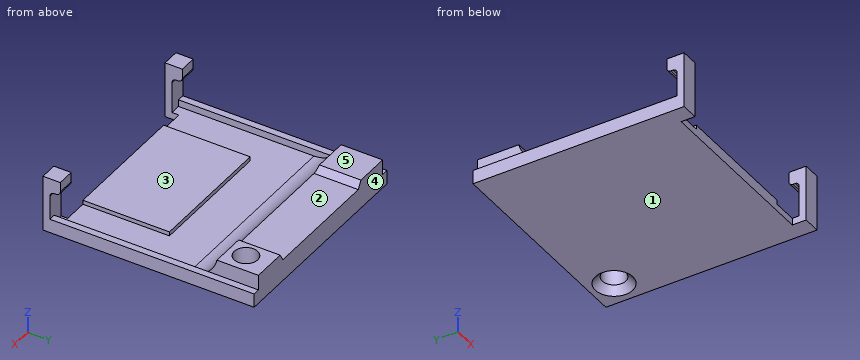
```python
from build123d import *

# Parameters (mm, degrees)
ESQUISSE1_W             = 28.6
ESQUISSE1_H             = 16.5
BOSS_EXTRU_1_DEPTH      = 1
ESQUISSE2_W             = 18.6
ESQUISSE2_H             = 12.5
BOSS_EXTRU_2_DEPTH      = 0.6
ESQUISSE3_W             = 28.6
ESQUISSE3_H             = 12
BOSS_EXTRU_3_DEPTH      = 1
ESQUISSE4_W             = 28.6
ESQUISSE4_H             = 6
BOSS_EXTRU_4_DEPTH      = 3.2
ESQUISSE5_R             = 1.7
ENL_V_MAT_EXTRU_1_DEPTH = 26.143438508
CONG_1_R                = 4
ESQUISSE6_W             = 1.5
ESQUISSE6_H             = 1
BOSS_EXTRU_5_DEPTH      = 2
ESQUISSE7_W             = 2.5
ESQUISSE7_H             = 1
BOSS_EXTRU_6_DEPTH      = 7.1
ESQUISSE8_W             = 2.5
ESQUISSE8_H             = 2
BOSS_EXTRU_7_DEPTH      = 1.5
CONG_2_R                = 0.6
ESQUISSE9_W             = 1
ESQUISSE9_H             = 30.5
BOSS_EXTRU_8_DEPTH      = 2
CHANFREIN2_SIZE         = 1
ENL_V_MAT_EXTRU_2_DEPTH = 10


with BuildPart() as part:
    # Esquisse1 → Boss.-Extru.1 (new body)
    with BuildSketch(Plane.XY):
        Rectangle(ESQUISSE1_W, ESQUISSE1_H)
    extrude(amount=BOSS_EXTRU_1_DEPTH)

    # Esquisse2 → Boss.-Extru.2 (add)
    with BuildSketch(Plane.XY.offset(1)):
        with Locations((0, -2)):
            Rectangle(ESQUISSE2_W, ESQUISSE2_H)
    extrude(amount=BOSS_EXTRU_2_DEPTH)

    # Esquisse3 → Boss.-Extru.3 (add)
    with BuildSketch(Plane(origin=(0, 0, 0), x_dir=(-1, 0, 0), z_dir=(0, 0, -1))):
        with Locations((0, 14.25)):
            Rectangle(ESQUISSE3_W, ESQUISSE3_H)
    extrude(amount=-BOSS_EXTRU_3_DEPTH)

    # Esquisse4 → Boss.-Extru.4 (add)
    with BuildSketch(Plane.XY.offset(1)):
        with Locations((0, 17.25)):
            Rectangle(ESQUISSE4_W, ESQUISSE4_H)
    extrude(amount=BOSS_EXTRU_4_DEPTH)

    # Esquisse5 → Enlèv. mat.-Extru.1 (cut, through all)
    with BuildSketch(Plane(origin=(0, 0, 0), x_dir=(-1, 0, 0), z_dir=(0, 0, -1))):
        with Locations((-11.6, 16.75)):
            Circle(ESQUISSE5_R)
    extrude(amount=-ENL_V_MAT_EXTRU_1_DEPTH, mode=Mode.SUBTRACT)

    # Congé1
    # the kernel refuses this fillet: 4 mm, written as the material it adds along each edge
    with BuildSketch(Plane(origin=(14.3, 14.25, 1), x_dir=(0, -1, 0), z_dir=(-1, 0, 0))) as cong_1_piece_1:
        with BuildLine():
            CenterArc((3.919183588, 4), CONG_1_R, 191.536959033, 78.463040967)
            Line((0, 3.2), (-0.078383672, 3.184))
            ThreePointArc((-0.078383672, 3.184), (-0.08, 1.6), (-0.08, 0))
            Line((-0.08, 0), (0, -0.08))
            Line((0, -0.08), (3.919183588, -0.08))
            Line((3.919183588, -0.08), (3.919183588, 0))
        make_face()
    extrude(amount=28.6)

    # Esquisse6 → Boss.-Extru.5 (add)
    with BuildSketch(Plane.XZ.offset(8.25)):
        with Locations((-13.55, 0.5)):
            Rectangle(ESQUISSE6_W, ESQUISSE6_H)
        with Locations((13.55, 0.5)):
            Rectangle(ESQUISSE6_W, ESQUISSE6_H)
    extrude(amount=BOSS_EXTRU_5_DEPTH)

    # Esquisse7 → Boss.-Extru.6 (add)
    with BuildSketch(Plane.XY.offset(1)):
        with Locations((-14.05, -9.75)):
            Rectangle(ESQUISSE7_W, ESQUISSE7_H)
        with Locations((14.05, -9.75)):
            Rectangle(ESQUISSE7_W, ESQUISSE7_H)
    extrude(amount=BOSS_EXTRU_6_DEPTH)

    # Esquisse8 → Boss.-Extru.7 (add)
    with BuildSketch(Plane(origin=(0, -9.25, 0), x_dir=(1, 0, 0), z_dir=(0, 1, 0))):
        with Locations((-14.05, -7.1)):
            Rectangle(ESQUISSE8_W, ESQUISSE8_H)
        with Locations((14.05, -7.1)):
            Rectangle(ESQUISSE8_W, ESQUISSE8_H)
    extrude(amount=BOSS_EXTRU_7_DEPTH)

    # Congé2
    cong_2_edges = [part.edges().sort_by_distance(p)[0] for p in [
        (-14.05, -9.25, 6.1),
        (-14.05, -7.75, 6.1),
        (14.05, -9.25, 6.1),
        (14.05, -7.75, 6.1),
    ]]
    fillet(cong_2_edges, radius=CONG_2_R)

    # Esquisse9 → Boss.-Extru.8 (add)
    with BuildSketch(Plane(origin=(0, 0, 0), x_dir=(-1, 0, 0), z_dir=(0, 0, -1))):
        with Locations((-14.8, 5)):
            Rectangle(ESQUISSE9_W, ESQUISSE9_H)
        with Locations((14.8, 5)):
            Rectangle(ESQUISSE9_W, ESQUISSE9_H)
    extrude(amount=-BOSS_EXTRU_8_DEPTH)

    # Chanfrein2
    chanfrein2_edges = [part.edges().sort_by_distance(p)[0] for p in [
        (13.3, 16.75, 0),
    ]]
    chamfer(chanfrein2_edges, length=CHANFREIN2_SIZE)

    # Esquisse10 → Enlèv. mat.-Extru.2 (cut)
    with BuildSketch(Plane(origin=(0, 20.25, 0), x_dir=(1, 0, 0), z_dir=(0, 1, 0))):
        Polygon((9.3, -4.2), (8.685937971, -3.136413366), (-8.685937971, -3.136413366), (-9.3, -4.2), align=None)
    extrude(amount=-ENL_V_MAT_EXTRU_2_DEPTH, mode=Mode.SUBTRACT)


solid = part.part
```
Read the model definition and answer for the solid it produces. Units are mm, in the model's axes. Face numbers are marked on the shaded views. A direction names the side the tool comes from. Coordinates: 2 decimals unless noted, no trailing zeros. Loops run counter-clockwise (first coordinate to the right, second up) from the corner with the lowest first, then second, coordinate; pieces in that order, holes last.
(1) Consider line 1 along Z through (x, y) = (0, 10.5); line 2 along X through (y, z) = (-9, 6.5); line 3 along Z through (x, y) = (-9, -7.5). Determine where each line is inside the solid, lowest interval first.
Solution:
line 1: z = 0 to 1
line 2: x = -15.3 to -12.8, 12.8 to 15.3
line 3: z = 0 to 1.6
(2) The mould has two halves that part along X. Classify the marked faces 1 and 2: released by +X, released by -X, zero draft, split by the parting line, or undercut.
Solution:
face 1: zero draft
face 2: undercut
(3) The part is cut by section A-A (x = 11.6). Determine the outline of the cut face in (y, z), and give its area (3 significant figures).
Solution:
outline: (-8.25, 0) - (14.05, 0) - (15.05, 1) - (15.05, 4.2) - (14.25, 4.2) arc R4 cw to (10.33, 1) - (-8.25, 1) - close; (18.45, 1) - (19.45, 0) - (20.25, 0) - (20.25, 4.2) - (18.45, 4.2) - close
area: 35.6 mm2
(4) A tool of negligible diameter and unlimited length cuts with its end or side. For the marked faces 3, 4 and 5, from which of +Z, -Z, +X, -X, +Y, -Y can it reach the whole face along a straight path? Write none if from no direction.
Solution:
face 3: +Z, -Y
face 4: +Z, -Z, +X, -X, +Y
face 5: +Z, +X, -X, +Y
(5) The part is cut by section B-B (z = 2.75). Determine the outline of the cut face in (x, y).
Solution:
outline: (-15.3, -10.25) - (-12.8, -10.25) - (-12.8, -9.25) - (-15.3, -9.25) - close; (-14.3, 13.64) - (14.3, 13.64) - (14.3, 20.25) - (-14.3, 20.25) - close; (12.8, -10.25) - (15.3, -10.25) - (15.3, -9.25) - (12.8, -9.25) - close; hole circle Ø3.4 at (11.6, 16.75)
(6) Flat-ended cylindrical pins translate along their axes: pin 1 Ø5.5 at (x, y) = (-11, 16.5) entering from +Z; pin 2 Ø6 at (x, y) = (-1, -4.5) entering from +Z; pin 3 Ø1.9 at (x, y) = (-2, 16.5) entering from +Z; pin 4 Ø2 at (x, y) = (11.6, 16.75) entering from -Z. Find the tip coordinate at first contact, or state that the pin passes through.
Solution:
pin 1: stops at z = 4.2
pin 2: stops at z = 1.6
pin 3: stops at z = 3.14
pin 4: passes through
(7) The part is cut by section C-C (y = 16.75). Determine the outline of the cut face in (x, z).
Solution:
outline: (-15.3, 0) - (8.9, 0) - (9.9, 1) - (9.9, 4.2) - (9.3, 4.2) - (8.69, 3.14) - (-8.69, 3.14) - (-9.3, 4.2) - (-14.3, 4.2) - (-14.3, 2) - (-15.3, 2) - close; (13.3, 1) - (14.3, 0) - (15.3, 0) - (15.3, 2) - (14.3, 2) - (14.3, 4.2) - (13.3, 4.2) - close
(8) The part is cut by section D-D (z = 5). Determine the outline of the cut face in (x, y).
Solution:
outline: (-15.3, -10.25) - (-12.8, -10.25) - (-12.8, -9.25) - (-15.3, -9.25) - close; (12.8, -10.25) - (15.3, -10.25) - (15.3, -9.25) - (12.8, -9.25) - close
